Autodesk Inventor part; units mm, degrees
ref_plane "YZ Plane" through (0, 0, 0) normal (1, 0, 0) x (0, 1, 0)
ref_plane "XZ Plane" through (0, 0, 0) normal (0, 1, 0) x (-1, 0, 0)
ref_plane "XY Plane" through (0, 0, 0) normal (0, 0, 1) x (1, 0, 0)
ref_plane "Arbeitsebene1" through (0, 0, 0) normal (0, 0, 1) x (1, 0, 0)
sketch "Skizze1" plane through (0, 0, 0) normal (0, 0, 1) x (1, 0, 0)
  circle A0 centre (-26.7746, 32.123) radius 1.5 construction
  circle A1 centre (15.7254, 11.123) radius 1.5 construction
  circle A2 centre (-26.2746, -24.877) radius 1.5 construction
  circle A3 centre (12.7254, -26.877) radius 1.5 construction
  circle A4 centre (12.7254, 30.123) radius 1.5 construction
  line L0 (11.0254, 3.323) -> (11.0254, -7.077) construction
  line L1 (11.0254, -7.077) -> (3.6254, -7.077) construction
  line L2 (3.6254, -7.077) -> (3.6254, 3.323) construction
  line L3 (3.6254, 3.323) -> (11.0254, 3.323) construction
  line L4 (3.6254, -32.077) -> (3.6254, -21.677) construction
  line L5 (3.6254, -21.677) -> (11.0254, -21.677) construction
  line L6 (11.0254, -21.677) -> (11.0254, -32.077) construction
  line L7 (11.0254, -32.077) -> (3.6254, -32.077) construction
  line L8 (11.0254, 27.923) -> (3.6254, 27.923) construction
  line L9 (3.6254, 27.923) -> (3.6254, 38.323) construction
  line L10 (3.6254, 38.323) -> (11.0254, 38.323) construction
  line L11 (11.0254, 38.323) -> (11.0254, 27.923) construction
  line L12 (-28.2746, 30.123) -> (-28.2746, -34.877) construction
  line L13 (-28.2746, -34.877) -> (-3.7746, -34.877) construction
  line L14 (-3.7746, -34.877) -> (-3.7746, -59.877) construction
  line L15 (-3.7746, -59.877) -> (10.8254, -59.877) construction
  line L16 (10.8254, -59.877) -> (10.8254, -34.877) construction
  line L17 (10.8254, -34.877) -> (20.2254, -34.877) construction
  line L18 (20.2254, -34.877) -> (20.2254, 39.123) construction
  line L19 (20.2254, 39.123) -> (10.8254, 39.123) construction
  line L20 (10.8254, 39.123) -> (10.8254, 49.123) construction
  line L21 (10.8254, 49.123) -> (-3.7746, 49.123) construction
  line L22 (-3.7746, 49.123) -> (-3.7746, 39.123) construction
  line L23 (-3.7746, 39.123) -> (-29.2746, 39.123) construction
  line L24 (-29.2746, 39.123) -> (-29.2746, 30.123) construction
  line L25 (-29.2746, 30.123) -> (-28.2746, 30.123) construction
  circle A5 centre (3.7254, 20.123) radius 7.5 construction
  line L26 (-3.7746, 49.123) -> (10.8254, 49.123) construction
  line L27 (10.8254, 49.123) -> (10.8254, -59.877) construction
  line L28 (10.8254, -59.877) -> (-3.7746, -59.877) construction
  line L29 (-3.7746, -59.877) -> (-3.7746, 49.123) construction
  line L30 (-3.7746, 49.123) -> (10.8254, 49.123)
  line L31 (10.8254, 49.123) -> (10.8254, -59.877)
  line L32 (10.8254, -59.877) -> (-3.7746, -59.877)
  line L33 (-3.7746, -59.877) -> (-3.7746, 49.123)
  circle A6 centre (3.7254, 44.123) radius 4.1
  circle A7 centre (3.7254, -53.877) radius 4.1
  line L34 (-8.2746, 32.123) -> (15.7254, 32.123)
  line L35 (15.7254, 32.123) -> (15.7254, 8.123)
  line L36 (15.7254, 8.123) -> (-8.2746, 8.123)
  line L37 (-8.2746, 8.123) -> (-8.2746, 32.123)
  line L38 (-8.2746, 32.123) -> (15.7254, 8.123) construction
  line L39 (15.7254, 32.123) -> (-8.2746, 8.123) construction
  circle A8 centre (3.7254, 20.123) radius 7.5
  circle A9 centre (3.7254, 20.123) radius 7.25
  line L40 (10.8254, 49.123) -> (10.9754, 49.123)
  line L41 (10.9754, 49.123) -> (10.9754, -59.877)
  line L42 (10.9754, -59.877) -> (10.8254, -59.877)
  line L43 (10.8254, -59.877) -> (10.8254, 49.123)
  point P0 (0, 0)
  dimension "d0" = 24
  dimension "d1" = 24
  dimension "d2" = 14.5
  dimension "d5" = 0.15
extrude "Extrusion1" add sketch "Skizze1" along normal blind 1 contours L30 L31 L34 L33 | L40 L41 L34 L31 | L34 L31 A8 L33 | L33 L36 L37 L34 | L34 L41 A8 L31 | A8 L31 L36 L33 | A8 L31 A9 | A8 L41 A9 L31 | L34 L35 L36 L41 A8 | L36 L31 L32 L33 | A8 L41 L36 L31 | L31 A9 L41 A8 | A9 L31 | A8 L41 | L36 L41 L42 L31 | A6 | A7 picked at (10.8531, 19.7957)
sketch "Skizze2" plane through (0, 0, 0) normal (0, 0, -1) x (-1, 0, 0)
  circle A0 centre (26.7746, 32.123) radius 1.5
  circle A1 centre (-15.7254, 11.123) radius 1.5
  circle A2 centre (26.2746, -24.877) radius 1.5
  circle A3 centre (-12.7254, -26.877) radius 1.5
  circle A4 centre (-12.7254, 30.123) radius 1.5
  line L0 (-11.0254, 3.323) -> (-11.0254, -7.077)
  line L1 (-11.0254, -7.077) -> (-3.6254, -7.077)
  line L2 (-3.6254, -7.077) -> (-3.6254, 3.323)
  line L3 (-3.6254, 3.323) -> (-11.0254, 3.323)
  line L4 (-3.6254, -32.077) -> (-3.6254, -21.677)
  line L5 (-3.6254, -21.677) -> (-11.0254, -21.677)
  line L6 (-11.0254, -21.677) -> (-11.0254, -32.077)
  line L7 (-11.0254, -32.077) -> (-3.6254, -32.077)
  line L8 (-11.0254, 27.923) -> (-3.6254, 27.923)
  line L9 (-3.6254, 27.923) -> (-3.6254, 38.323)
  line L10 (-3.6254, 38.323) -> (-11.0254, 38.323)
  line L11 (-11.0254, 38.323) -> (-11.0254, 27.923)
  line L12 (28.2746, 30.123) -> (28.2746, -34.877)
  line L13 (28.2746, -34.877) -> (3.7746, -34.877)
  line L14 (3.7746, -34.877) -> (3.7746, -59.877)
  line L15 (3.7746, -59.877) -> (-10.8254, -59.877)
  line L16 (-10.8254, -59.877) -> (-10.8254, -34.877)
  line L17 (-10.8254, -34.877) -> (-20.2254, -34.877)
  line L18 (-20.2254, -34.877) -> (-20.2254, 39.123)
  line L19 (-20.2254, 39.123) -> (-10.8254, 39.123)
  line L20 (-10.8254, 39.123) -> (-10.8254, 49.123)
  line L21 (-10.8254, 49.123) -> (3.7746, 49.123)
  line L22 (3.7746, 49.123) -> (3.7746, 39.123)
  line L23 (3.7746, 39.123) -> (29.2746, 39.123)
  line L24 (29.2746, 39.123) -> (29.2746, 30.123)
  line L25 (29.2746, 30.123) -> (28.2746, 30.123)
  circle A5 centre (-3.7254, 20.123) radius 7.5
  line L26 (-3.8254, 38.123) -> (-3.8254, 28.123)
  line L27 (-3.8254, 28.123) -> (-10.8254, 28.123)
  line L28 (-10.8254, 28.123) -> (-10.8254, 38.123)
  line L29 (-10.8254, 38.123) -> (-3.8254, 38.123)
  line L30 (-3.8254, 3.123) -> (-3.8254, -6.877)
  line L31 (-3.8254, -6.877) -> (-10.8254, -6.877)
  line L32 (-10.8254, -6.877) -> (-10.8254, 3.123)
  line L33 (-10.8254, 3.123) -> (-3.8254, 3.123)
  line L34 (-10.8254, -21.877) -> (-3.8254, -21.877)
  line L35 (-3.8254, -21.877) -> (-3.8254, -31.877)
  line L36 (-3.8254, -31.877) -> (-10.8254, -31.877)
  line L37 (-10.8254, -31.877) -> (-10.8254, -21.877)
  point P0 (0, 0)
  dimension "d7" = 0.2
  dimension "d8" = 0.2
  dimension "d9" = 0.2
extrude "Extrusion2" add sketch "Skizze2" along normal blind 1 contours L26 L27 L28 L29 | L30 L31 L32 L33 | L34 L35 L36 L37
sketch "Skizze3" plane through (0, 0, 1) normal (0, 0, 1) x (1, 0, 0)
  circle A0 centre (3.7254, 20.123) radius 3.5 construction
  arc A1 (-0.3746, 17.023) -> (0.6254, 16.023) centre (0.6254, 17.023) ccw construction
  line L0 (0.6254, 16.023) -> (6.8254, 16.023) construction
  arc A2 (6.8254, 16.023) -> (7.8254, 17.023) centre (6.8254, 17.023) ccw construction
  line L1 (7.8254, 17.023) -> (7.8254, 18.7249) construction
  line L2 (7.8254, 18.7249) -> (9.8254, 18.7249) construction
  line L3 (9.8254, 19.2249) -> (9.8254, 18.7249) construction
  line L4 (7.8254, 19.2249) -> (9.8254, 19.2249) construction
  line L5 (7.8254, 19.2249) -> (7.8254, 21.021) construction
  line L6 (7.8254, 21.021) -> (9.8254, 21.021) construction
  line L7 (9.8254, 21.521) -> (9.8254, 21.021) construction
  line L8 (7.8254, 21.521) -> (9.8254, 21.521) construction
  line L9 (7.8254, 21.521) -> (7.8254, 23.223) construction
  arc A3 (7.8254, 23.223) -> (6.8254, 24.223) centre (6.8254, 23.223) ccw construction
  line L10 (6.8254, 24.223) -> (0.6254, 24.223) construction
  arc A4 (0.6254, 24.223) -> (-0.3746, 23.223) centre (0.6254, 23.223) ccw construction
  line L11 (-0.3746, 23.223) -> (-0.3746, 17.023) construction
  line L12 (10.9754, 49.123) -> (-3.7746, 49.123)
  line L13 (-3.7746, 49.123) -> (-3.7746, 32.123)
  line L14 (-3.7746, 32.123) -> (-8.2746, 32.123)
  line L15 (-8.2746, 32.123) -> (-8.2746, 8.123)
  line L16 (-8.2746, 8.123) -> (-3.7746, 8.123)
  line L17 (-3.7746, 8.123) -> (-3.7746, -59.877)
  line L18 (-3.7746, -59.877) -> (10.9754, -59.877)
  line L19 (10.9754, -59.877) -> (10.9754, 8.123)
  line L20 (10.9754, 8.123) -> (15.7254, 8.123)
  line L21 (15.7254, 8.123) -> (15.7254, 32.123)
  line L22 (15.7254, 32.123) -> (10.9754, 32.123)
  line L23 (10.9754, 32.123) -> (10.9754, 49.123)
  circle A5 centre (3.7254, 44.123) radius 4.1
  circle A6 centre (3.7254, -53.877) radius 4.1
  line L24 (-0.3246, 18.4454) -> (-0.3246, 21.8005)
  line L25 (-0.3246, 21.8005) -> (2.0478, 24.173)
  line L26 (2.0478, 24.173) -> (5.403, 24.173)
  line L27 (5.403, 24.173) -> (7.7754, 21.8005)
  line L28 (7.7754, 21.8005) -> (7.7754, 18.4454)
  line L29 (7.7754, 18.4454) -> (5.403, 16.073)
  line L30 (5.403, 16.073) -> (2.0478, 16.073)
  line L31 (2.0478, 16.073) -> (-0.3246, 18.4454)
  line L32 (-8.2746, 32.123) -> (-8.2746, 8.123)
  point P0 (0, 0)
  dimension "d16" = 8.1
extrude "Extrusion3" add sketch "Skizze3" along normal blind 1.8
properties part number "02_Lensadapter"
The listing builds one solid part. Answer for the finished solid, in the listing's coordinates (mm). A direction names the side the tool comes from. Coordinates: 2 decimals unless noted, no trailing zeros. Loops run counter-clockwise (first coordinate to the right, second up) from the corner with the lowest first, then second, coordinate; pieces in that order, holes last. Notation, with made-up numbers: (-31.5, -31.75) - (25.5, -31.75) arc R29 ccw to (25.5, -5.75) - close; hole circle Ø10 at (83, 18). An arc over 180 degrees is marked (long way). Use a Markdown table: item, result. Add a question column.
1) Find the intervals of material crossed by line 1 (Y direction, x = 7, z = 1.85); line 2 (Y direction, x = 5.25, z = 1.05); line 3 (X direction, y = 5, z = 0.05), in increasing order.
2) Given pin 1 (2 mm diameter, centred on y = -24, z = 2, fed in from -X); pin 2 (10.5 mm diameter, centred on x = 3.73, y = 44.12, fed in from +Z); pin 3 (0.8 mm diameter, centred on x = 7.5, z = -0.5, fed in from -Y); pin 4 (1.5 mm diameter, centred on x = -5.5, z = 1, fed in from +Y), each flat-ended and moving along its own axis, determine where each tip first touches the part or whether it passes through.
3) The part is cut by section D-D, the plane y = 41. Give the vertices of the cut face in (x, z), and give its area (3 significant figures).
4) The part is cut by section C-C, the plane x = -5.5. Give the vertices of the cut face in (y, z).
5) The part is cut by section B-B, the plane z = 1.85. Give the vertices of the cut face in (x, y), and give its area (3 significant figures).
6) For faces 1 (the flat face through (7.775, 20, 2)), 2 (the flat face through (13, 8.123, 1)), 3 (the flat face through (4, 44, 1)), determine the directions among +Z, -Z, +X, -X, +Y, -Y from which every point of the face is accessible in a straight line to the end or side of a thin tool.
7) The part is cut by section A-A, the plane y = 2. Give the vertices of the cut face in (x, z).
8) The mould has two halves that part along X. Classify faces 4 (the flat face through (7, 17, 1)), 5 (the flat face through (13, 32.123, 1)), 6 (the flat face through (-8.275, 20, 1)): released by +X, released by -X, zero draft, split by the parting line, or undercut.
Here are the results:
| question | item | result |
|---|---|---|
| 1 | line 1 | y = -59.88 to -56.34, -51.41 to 17.67, 22.58 to 41.66, 46.59 to 49.12 |
| 1 | line 2 | y = -59.88 to -57.68, -50.07 to 16.07, 24.17 to 40.32, 47.93 to 49.12 |
| 1 | line 3 | x = -3.77 to 10.98 |
| 2 | pin 1 | stops at x = -3.77 |
| 2 | pin 2 | stops at z = 2.8 |
| 2 | pin 3 | stops at y = -31.88 |
| 2 | pin 4 | stops at y = 32.12 |
| 3 | outline | (-3.77, 0) - (10.98, 0) - (10.98, 2.8) - (6.38, 2.8) - (6.38, 1) - (1.07, 1) - (1.07, 2.8) - (-3.77, 2.8) - close |
| 3 | area | 31.7 mm^2 |
| 4 | outline | (8.12, 0) - (32.12, 0) - (32.12, 2.8) - (8.12, 2.8) - close |
| 5 | outline | (-8.27, 8.12) - (-3.77, 8.12) - (-3.77, -59.88) - (10.98, -59.88) - (10.98, 8.12) - (15.73, 8.12) - (15.73, 32.12) - (10.98, 32.12) - (10.98, 49.12) - (-3.77, 49.12) - (-3.77, 32.12) - (-8.27, 32.12) - close; hole circle Ø8.2 at (3.73, -53.88); hole circle Ø8.2 at (3.73, 44.12); hole (-0.32, 18.45) - (2.05, 16.07) - (5.4, 16.07) - (7.78, 18.45) - (7.78, 21.8) - (5.4, 24.17) - (2.05, 24.17) - (-0.32, 21.8) - close |
| 5 | area | 1,670 mm^2 |
| 6 | face 1 | +Z, -Z |
| 6 | face 2 | +Z, -Z, +X, -Y |
| 6 | face 3 | +Z |
| 7 | outline | (-3.77, 0) - (3.83, 0) - (3.83, -1) - (10.83, -1) - (10.83, 0) - (10.98, 0) - (10.98, 2.8) - (-3.77, 2.8) - close |
| 8 | face 4 | undercut |
| 8 | face 5 | zero draft |
| 8 | face 6 | released by -X |
